Could you check a few things on this model? Use its own coordinates, in mm. A direction names the side the tool comes from. Coordinates: 2 decimals unless noted, no trailing zeros. Loops run counter-clockwise (first coordinate to the right, second up) from the corner with the lowest first, then second, coordinate; pieces in that order, holes last. Notation, with made-up numbers: (-19, 44) - (28, 44) arc R19 ccw to (28, 72) - close; hole circle Ø6 at (-27.75, -7). An arc over 180 degrees is marked (long way). Put each result on its own line as item: value. Start each with the question number.
```python
from build123d import *

# Parameters (mm, degrees)
SKETCH_W        = 72.5
SKETCH_H        = 21.5
PAD_DEPTH       = 17
SKETCH001_W     = 52.7
SKETCH001_H     = 17.7
POCKET_DEPTH    = 15
SKETCH002_W     = 48.2
SKETCH002_H     = 13.2
POCKET001_DEPTH = 5
SKETCH003_W     = 10
SKETCH003_H     = 28.534706
SKETCH003_W_2   = 11.202904
SKETCH003_H_2   = 28.537951
POCKET002_DEPTH = 14
SKETCH004_R     = 1.7
POCKET003_DEPTH = 5
SKETCH005_W     = 12
SKETCH005_H     = 2
PAD001_DEPTH    = 1
FILLET_R        = 0.99
FILLET001_R     = 3
FILLET002_R     = 3


with BuildPart() as part:
    # Sketch → Pad (new body)
    with BuildSketch(Plane.XY):
        Rectangle(SKETCH_W, SKETCH_H)
    extrude(amount=PAD_DEPTH)

    # Sketch001 → Pocket (cut)
    with BuildSketch(Plane.XY.offset(17)):
        Rectangle(SKETCH001_W, SKETCH001_H)
    extrude(amount=-POCKET_DEPTH, mode=Mode.SUBTRACT)

    # Sketch002 → Pocket001 (cut)
    with BuildSketch(Plane.XY.offset(2)):
        Rectangle(SKETCH002_W, SKETCH002_H)
    extrude(amount=-POCKET001_DEPTH, mode=Mode.SUBTRACT)

    # Sketch003 → Pocket002 (cut)
    with BuildSketch(Plane(origin=(0, 0, 0), x_dir=(1, 0, 0), z_dir=(0, 0, -1))):
        with Locations((-33, -0.267353)):
            Rectangle(SKETCH003_W, SKETCH003_H)
        with Locations((33.601452, -0.268975)):
            Rectangle(SKETCH003_W_2, SKETCH003_H_2)
    extrude(amount=-POCKET002_DEPTH, mode=Mode.SUBTRACT)

    # Sketch004 → Pocket003 (cut)
    with BuildSketch(Plane(origin=(0, 0, 14), x_dir=(1, 0, 0), z_dir=(0, 0, -1))):
        with Locations((32, 0)):
            Circle(SKETCH004_R)
        with Locations((-32, 0)):
            Circle(SKETCH004_R)
    extrude(amount=-POCKET003_DEPTH, mode=Mode.SUBTRACT)

    # Sketch005 → Pad001 (new body)
    with BuildSketch(Plane(origin=(0, -8.85, 0), x_dir=(-1, 0, 0), z_dir=(0, 1, 0))):
        with Locations((0, 14.2)):
            Rectangle(SKETCH005_W, SKETCH005_H)
    extrude(amount=PAD001_DEPTH)

    # Fillet
    fillet_edges = [part.edges().sort_by_distance(p)[0] for p in [
        (0, -7.85, 15.2),
        (0, -7.85, 13.2),
    ]]
    fillet(fillet_edges, radius=FILLET_R)

    # Fillet001
    fillet001_edges = [part.edges().sort_by_distance(p)[0] for p in [
        (36.25, 10.75, 15.5),
        (36.25, -10.75, 15.5),
        (-36.25, 10.75, 15.5),
        (-36.25, -10.75, 15.5),
    ]]
    fillet(fillet001_edges, radius=FILLET001_R)

    # Fillet002
    fillet002_edges = [part.edges().sort_by_distance(p)[0] for p in [
        (0, -10.75, 0),
        (-28, 0, 0),
        (0, 10.75, 0),
        (28, 0, 0),
        (28, 10.75, 7),
        (28, -10.75, 7),
        (-28, -10.75, 7),
        (-28, 10.75, 7),
    ]]
    fillet(fillet002_edges, radius=FILLET002_R)


solid = part.part
```
(1) For pin 1 Ø3 at (x, y) = (-4, 4.5) entering from -Z; pin 2 Ø3.5 at (y, z) = (-2, 8.5) entering from -X; pin 3 Ø3.5 at (x, y) = (-31, -4) entering from -Z; pin 4 Ø2 at (x, z) = (-5.5, 1) entering from -Y, each with a flat end and sliding along its axis, tell me the tip position at first contact or that it passes through.
(2) I need wall thicknesses on L1, parallel to X at y = 0, z = 15.7; L2, parallel to Y at x = 32, z = 15.3; L3, parallel to X at y = -3.25, z = 4. Which ranges of each line are inside material? Lowest first, please. Write a range as [from, to].
(3) I want a section at A-A on y = 0. List the corners of the cut face in (x, z) for me, and give its area (3 significant figures).
(4) If we mould it in two halves opening along X, with no side actions, what happens to faces 1 (the flat face through (36.25, 0, 15)), 2 (the flat face through (-24.1, 0, 1)), 3 (the cylindrical face through (-27.14, -0.11, 0.9))? For each: pulls with the +X half, pulls with the -X half, needs draft (parallel to the pull), parting line crosses it, or undercut.
(5) Which directions (+Z, -Z, +X, -X, +Y, -Y) give clear straight access to the entire face, cutting with the end or side of a thin tool? Please do faces 4 (the cylindrical face through (-27.1, -9.89, 8.42)), 5 (the flat face through (0, 6.6, 1)), 6 (the flat face through (26.35, 0, 10)), 7 (the cylindrical face through (-27.1, 9.89, 8.42)).
(6) I want a section at B-B on x = -23. List the corners of the cut face in (y, z) for me, and give its area (3 significant figures).
(7) I want a section at D-D on z = 3.75. List the corners of the cut face in (x, y) for me, and give its area (3 significant figures).
(8) I want a section at C-C on y = 2.75. List the corners of the cut face in (x, z) for me.
Answer sheet:
1. pin 1: passes through
1. pin 2: stops at x = -28
1. pin 3: stops at z = 14
1. pin 4: stops at y = -10.58
2. L1: x = [-36.25, -33.7], [-30.3, -26.35], [26.35, 30.3], [33.7, 36.25]
2. L2: y = [-10.75, -1.7], [1.7, 10.75]
2. L3: x = [-28, -26.35], [26.35, 28]
3. outline: (-36.25, 14) - (-33.7, 14) - (-33.7, 17) - (-36.25, 17) - close; (-30.3, 14) - (-28, 14) - (-28, 3) arc R3 ccw to (-25, 0) - (-24.1, 0) - (-24.1, 2) - (-26.35, 2) - (-26.35, 17) - (-30.3, 17) - close; (24.1, 0) - (25, 0) arc R3 ccw to (28, 3) - (28, 14) - (30.3, 14) - (30.3, 17) - (26.35, 17) - (26.35, 2) - (24.1, 2) - close; (33.7, 14) - (36.25, 14) - (36.25, 17) - (33.7, 17) - close
3. area: 90.3 mm^2
4. face 1: pulls with the +X half
4. face 2: undercut
4. face 3: pulls with the -X half
5. face 4: -Z, -X, -Y
5. face 5: +Z, -Z
5. face 6: +Z
5. face 7: -Z, -X, +Y
6. outline: (-10.75, 3) arc R3 ccw to (-7.75, 0) - (-6.6, 0) - (-6.6, 2) - (-8.85, 2) - (-8.85, 17) - (-10.75, 17) - close; (6.6, 0) - (7.75, 0) arc R3 ccw to (10.75, 3) - (10.75, 17) - (8.85, 17) - (8.85, 2) - (6.6, 2) - close
6. area: 69.7 mm^2
7. outline: (-28, -7.75) arc R3 ccw to (-25, -10.75) - (25, -10.75) arc R3 ccw to (28, -7.75) - (28, 7.75) arc R3 ccw to (25, 10.75) - (-25, 10.75) arc R3 ccw to (-28, 7.75) - close; hole (-26.35, -8.85) - (26.35, -8.85) - (26.35, 8.85) - (-26.35, 8.85) - close
7. area: 263 mm^2
8. outline: (-36.25, 14) - (-28, 14) - (-28, 3) arc R3 ccw to (-25, 0) - (-24.1, 0) - (-24.1, 2) - (-26.35, 2) - (-26.35, 17) - (-36.25, 17) - close; (24.1, 0) - (25, 0) arc R3 ccw to (28, 3) - (28, 14) - (36.25, 14) - (36.25, 17) - (26.35, 17) - (26.35, 2) - (24.1, 2) - close
